Print and shaded views of the part. All mm, measured from the part's lowest x, y and z. Round coordinates to 2 decimals unless told otherwise and drop trailing zeros. Loops run counter-clockwise (first coordinate to the right, second up) from the corner with the lowest first, then second, coordinate; pieces in that order, holes last. Notation, with made-up numbers: (18, 48) - (22, 48) arc R31 ccw to (22, 83) - close; hole circle Ø7 at (-25, 80). An arc over 180 degrees is marked (long way). Use one line per item in the form item = value.
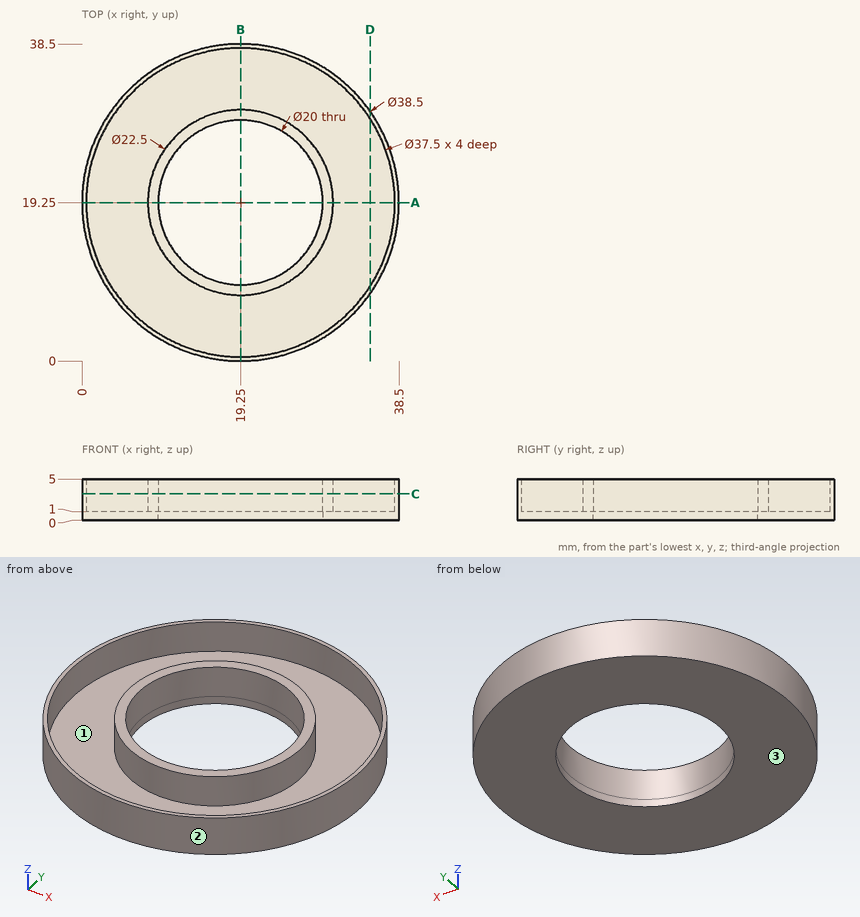
1) Slice it at D-D (x = 35). Write the cut outline in (y, z), plus the area to 3 significant figures.
Report:
outline = (8.18, 0) - (30.32, 0) - (30.32, 5) - (29.42, 5) - (29.42, 1) - (9.08, 1) - (9.08, 5) - (8.18, 5) - close
area = 29.3 mm^2
2) Slice it at C-C (z = 3.2). Write the cut outline in (x, y), plus the area to 3 significant figures.
Report:
outline = circle Ø38.5 at (19.25, 19.25); circle Ø22.5 at (19.25, 19.25); hole circle Ø37.5 at (19.25, 19.25); hole circle Ø20 at (19.25, 19.25)
area = 143 mm^2
3) Two-plate mould, pull along Y, no slides. Class the marked faces 1, 2 and 3: +Y half, -Y half, draft (parallel to the pull), parting line (faces both ways), or undercut.
Report:
face_1 = undercut
face_2 = parting line
face_3 = draft
4) Drill centre lines: probe 1 along Y at (x, z) = (19.25, 3.5); probe 2 along Y at (x, z) = (15, 4.35); probe 3 along X at (y, z) = (13, 1.7). Where is each one in solid material? Low to high.
Report:
probe_1 = 0 to 0.5, 8 to 9.25, 29.25 to 30.5, 38 to 38.5
probe_2 = 0.48 to 0.99, 8.83 to 10.2, 28.3 to 29.67, 37.51 to 38.02
probe_3 = 1.04 to 1.57, 9.9 to 11.44, 27.06 to 28.6, 36.93 to 37.46
5) Flat gauge pins, fed straight in: pin 1 (12 mm diameter, centred on x = 19.25, y = 19.25, fed in from -Z); pin 2 (5 mm diameter, centred on x = 5.5, y = 17, fed in from +Z); pin 3 (1 mm diameter, centred on y = 28, z = 1, fed in from -X); pin 4 (1 mm diameter, centred on x = 31, z = 2, fed in from +Y). Where does each tip first touch, or does it go through?
Report:
pin_1 = through
pin_2 = 1
pin_3 = 1.86
pin_4 = 34.87
6) Slice it at A-A (y = 19.25). Write the cut outline in (x, z).
Report:
outline = (0, 0) - (9.25, 0) - (9.25, 5) - (8, 5) - (8, 1) - (0.5, 1) - (0.5, 5) - (0, 5) - close; (29.25, 0) - (38.5, 0) - (38.5, 5) - (38, 5) - (38, 1) - (30.5, 1) - (30.5, 5) - (29.25, 5) - close
